```python
from build123d import *

# Parameters (mm, degrees)
F1_DEPTH = 20
F2_R     = 5
F4_DEPTH = 25


with BuildPart() as f1:
    # F0 (on Top) → F1 (new body)
    with BuildSketch(Plane.XY):
        with BuildLine():
            Line((0, 37.5), (0, 50))
            ThreePointArc((0, 50), (-35.355339, 35.355339), (-50, 0))
            Line((-50, 0), (-37.5, 0))
            ThreePointArc((-37.5, 0), (-26.516504, 26.516504), (0, 37.5))
        make_face()
    extrude(amount=F1_DEPTH)

    # F2
    f2_edges = [f1.edges().sort_by_distance(p)[0] for p in [
        (-26.516504, 26.516504, 0),
        (-26.516504, 26.516504, 20),
        (-43.75, 0, 0),
        (-43.75, 0, 20),
        (0, 43.75, 0),
        (0, 43.75, 20),
        (-50, 0, 10),
        (0, 50, 10),
        (0, 37.5, 10),
        (-37.5, 0, 10),
        (-35.355339, 35.355339, 0),
        (-35.355339, 35.355339, 20),
    ]]
    fillet(f2_edges, radius=F2_R)

    # F3 (on face) → F4 (join)
    with BuildSketch(Plane.XY.offset(20)):
        Polygon((-5, 44.72136), (-44.72136, 5), (-42.204858, 5), (-5, 42.204858), align=None)
    extrude(amount=F4_DEPTH)


solid = f1.part
```
Part model, mm, in its own coordinate system. A direction names the side the tool comes from. Give positions to 0.01 mm unless a question says otherwise; leave off trailing zeros. Order: outer loops, then holes, each group sorted by start corner. A loop starts at its lowest first (then second) coordinate and runs counter-clockwise, first axis right, second up. Notation, with made-up numbers: M 88,-16 L 108,-16 A13 cw 108,1 Z; hole C 9,-12.5 d8. An arc over 180 degrees is marked long. Use a Markdown table: item, result. Add a question column.
(1) Saw through at B-B, the plane z = 23.5. Give the cut face in (x, y).
(2) Probe line 1 along Z through (x, y) = (-13, 43.5); line 2 along X through (y, z) = (42.5, 24); line 3 along X through (y, z) = (10, 30). List the from-to ranges inside material, lowest first. Write a range as [from, to].
(3) Saw through at C-C, the plane z = 4. Give the cut face in (x, y).
(4) Saw through at A-A, the plane z = 12. Give the cut face in (x, y), and give its area (3 significant figures).
(5) 3-axis set-ups, long thin cutter, end or side, ignore diameter. For faces 1 (the face through (-43, 5, 32)), 2 (the face through (-26.76, 26.27, 9.93)), 3 (the face through (-5, 43, 32)): which of +Z, -Z, +X, -X, +Y, -Y reach the whole face in a straight line?
(6) Mould opens along Z. For faces 4 (the face through (-1, 43, 2)), 5 (the face through (-24, 24, 20)), 6 (the face through (-35.02, 35.69, 9.93)) say: +Z half, -Z half, draft (parallel to the pull), parting line (faces both ways), or undercut.
(7) Drop flat-ended pins along their axis: P1, Ø3, axis at y = 7, z = 19, coming from the +X side; P2, Ø10, axis at y = 20, z = 15.5, coming from the -X side; P3, Ø10, axis at y = 17.5, z = 38, coming from the -X side. Give the stop position or say it passes through.
Answer key:
| question | item | result |
|---|---|---|
| 1 | outline | M -44.72,5 L -42.2,5 L -5,42.2 L -5,44.72 Z |
| 2 | line 1 | [0.02, 19.98] |
| 2 | line 2 | [-7.22, -5] |
| 2 | line 3 | [-39.72, -37.2] |
| 3 | outline | M -49.59,5.54 A4.9 ccw -44.72,0.1 L -42.2,0.1 A4.9 ccw -37.34,4.42 A37.6 cw -4.42,37.34 A4.9 ccw -0.1,42.2 L -0.1,44.72 A4.9 ccw -5.54,49.59 A49.9 ccw Z |
| 4 | outline | M -49.69,5.56 A5 ccw -44.72,0 L -42.2,0 A5 ccw -37.24,4.41 A37.5 cw -4.41,37.24 A5 ccw 0,42.2 L 0,44.72 A5 ccw -5.56,49.69 A50 ccw Z |
| 4 | area | 837 mm^2 |
| 5 | face 1 | +Z, +X, -X, -Y |
| 5 | face 2 | -Z, +X, -Y |
| 5 | face 3 | +Z, +X, +Y, -Y |
| 6 | face 4 | -Z half |
| 6 | face 5 | undercut |
| 6 | face 6 | draft |
| 7 | P1 | x = -37.48 |
| 7 | P2 | x = -47.69 |
| 7 | P3 | x = -37.22 |
